Input: part model. Units: mm. Frame: model coordinates. A direction names the side the tool comes from. Coordinates: 2 decimals unless noted, no trailing zeros. Order: outer loops, then holes, each group sorted by start corner. A loop starts at its lowest first (then second) coordinate and runs counter-clockwise, first axis right, second up. Notation, with made-up numbers: (58, 47.5) -> (96, 47.5) arc R23 ccw to (96, 77.5) -> close; hole circle Ø7 at (24.5, 84). An arc over 180 degrees is marked (long way). Use one line per item in the form item = value. Start each with the question number.
1) Section query C-C on x = 8. Output: boundary loops of the cut face in (y, z).
2) Access query for faces 4 (the flat face through (25, -10, 17)), 5 (the flat face through (-48, 12, 10)), 6 (the flat face through (-62, -12, 2)), 7 (the flat face through (-31, -33, 71)), 8 (the flat face through (-46.22, -25.416, 19.564)). Directions: +Z, -Z, +X, -X, +Y, -Y. A direction counts if a zero-diameter tool reaches every point of the face in a straight line with its end or side. Return the directions, or none.
3) Draft query along X for faces 1 (the flat face through (-62, -19.5, 75)), 2 (the flat face through (-29, -33, 71)), 3 (the flat face through (-78.73, 3.11, 20.14)). Return one class per face: pulls with the +X half, pulls with the -X half, needs draft (parallel to the pull), parting line crosses it, or undercut.
4) Section query A-A on y = 8. Output: boundary loops of the cut face in (x, z).
5) Section query B-B on y = -8. Output: boundary loops of the cut face in (x, z), then the cut area to 3 significant figures.
6) Ray query, line 1 along Y through (x, z) = (0, 27); line 2 along X through (y, z) = (0.5, 56); line 3 along X through (y, z) = (-8, 4). Return the intervals inside material, ascending.
7) Pin query (flat end, axial travel): pin 1 (1.1 mm diameter, centred on y = -34, z = 11, fed in from +X); pin 2 (10 mm diameter, centred on x = 7.5, y = -12, fed in from +Z); pin 3 (13 mm diameter, centred on y = -7.5, z = 65.5, fed in from +X); pin 4 (2.5 mm diameter, centred on x = 8, y = 0, fed in from -Z). Return the tip coordinate at first contact, or that it passes through.
8) Section query D-D on y = -16. Output: boundary loops of the cut face in (x, z).
from build123d import *
from build123d.topology import SkipClean

# Parameters (mm, degrees)
SKETCH_1_W            = 50
SKETCH_1_H            = 35
EXTRUDE_1_DEPTH       = 10
HOLE_WIZARD_370_D     = 10.5
HOLE_WIZARD_475_D     = 3.2
SKETCH_6_W            = 10
SKETCH_6_H            = 52
EXTRUDE_2_DEPTH       = 70
EXTRUDE_3_DEPTH       = 52
SKETCH_10_W           = 30
SKETCH_10_H           = 15
SKETCH_10_H_2         = 7
CUT_EXTRUDE_1_DEPTH   = 66
SKETCH_12_W           = 5
SKETCH_12_H           = 15
EXTRUDE_4_DEPTH       = 2
EXTRUDE_5_DEPTH       = 10
RIB_6_REACH           = 107.429
SKETCH_15_WALL_W      = 243.090204886
SKETCH_15_WALL_H      = 10
SKETCH_16_W           = 10
SKETCH_16_H           = 10
EXTRUDE_6_DEPTH       = 17
FILLET_1_RADIUS       = 5
FILLET_1_LENGTH       = 10
CUT_EXTRUDE_3_DEPTH   = 3
EXTRUDE_8_DEPTH       = 2
FILLET_3_R            = 1
SKETCH_20_R           = 5
CUT_EXTRUDE_4_DEPTH   = 106.654483654
CHAMFER_3_SIZE        = 3
SKETCH_22_R           = 1.6
SKETCH_22_R_2         = 4.65
SKETCH_22_R_3         = 5.25
EXTRUDE_9_DEPTH       = 74
EXTRUDE_10_DEPTH      = 49
SKETCH_25_W           = 30
SKETCH_25_H           = 15
CUT_EXTRUDE_5_DEPTH   = 66
SKETCH_26_R           = 12.5
CUT_EXTRUDE_6_DEPTH   = 50
SKETCH_27_W           = 25
SKETCH_27_H           = 70.37051412
SKETCH_27_W_2         = 27.110275364
CUT_EXTRUDE_7_DEPTH   = 50
SKETCH_28_R           = 5
CUT_EXTRUDE_8_DEPTH   = 132.601177488
MIRROR_2_COPY_1_DEPTH = 2


with BuildPart() as part:
    # 草图1 → 凸台-拉伸1 (new body)
    with BuildSketch(Plane.XY):
        Rectangle(SKETCH_1_W, SKETCH_1_H)
    extrude(amount=EXTRUDE_1_DEPTH)

    # Hole Wizard 370 (through all)
    with Locations(Plane.XY.offset(10)):
        with Locations((0, 0)):
            Hole(HOLE_WIZARD_370_D / 2)

    # Hole Wizard 475 (through all)
    with Locations(Plane.XY.offset(10)):
        with Locations((8, 0), (0, 8), (-8, 0), (0, -8)):
            Hole(HOLE_WIZARD_475_D / 2)

    # 草图6 → 凸台-拉伸2 (add)
    with BuildSketch(Plane.ZY.offset(25)):
        with Locations((5, -8.5)):
            Rectangle(SKETCH_6_W, SKETCH_6_H)
    extrude(amount=EXTRUDE_2_DEPTH)

    # 草图9 → 凸台-拉伸3 (add, through all)
    with BuildSketch(Plane(origin=(0, 17.5, 0), x_dir=(1, 0, 0), z_dir=(0, 1, 0))):
        Polygon((-95, -30), (-62, -10), (-95, -10), align=None)
        Polygon((-29, -30), (-29, -10), (-62, -10), align=None)
    extrude(amount=-EXTRUDE_3_DEPTH)

    # 草图10 → 切除-拉伸1 (cut)
    with BuildSketch(Plane.ZY.offset(95)):
        with Locations((15, -12)):
            Rectangle(SKETCH_10_W, SKETCH_10_H)
        with Locations((15, 14)):
            Rectangle(SKETCH_10_W, SKETCH_10_H_2)
    extrude(amount=-CUT_EXTRUDE_1_DEPTH, mode=Mode.SUBTRACT)

    # 草图12 → 凸台-拉伸4 (add)
    with BuildSketch(Plane(origin=(0, 0, 0), x_dir=(-1, 0, 0), z_dir=(0, 0, -1))):
        with Locations((85.5, -12)):
            Rectangle(SKETCH_12_W, SKETCH_12_H)
        with Locations((39.5, -12)):
            Rectangle(SKETCH_12_W, SKETCH_12_H)
        with Locations((62.5, -12)):
            Rectangle(SKETCH_12_W, SKETCH_12_H)
    extrude(amount=-EXTRUDE_4_DEPTH)

    # 草图14 → 凸台-拉伸5 (add)
    with BuildSketch(Plane(origin=(0, 0, 0), x_dir=(-1, 0, 0), z_dir=(0, 0, -1))):
        Polygon((95, 10.5), (29, 17.5), (29, 10.5), align=None)
    extrude(amount=-EXTRUDE_5_DEPTH)

    # 草图15 wall → 筋6 (add, up to next)
    with BuildSketch(Plane(origin=(-12.5, -26, 0), x_dir=(0.82692650207, 0.562310021407, 0), z_dir=(0.562310021407, -0.82692650207, 0)), mode=Mode.PRIVATE) as rib_6_sk1:
        with Locations((0, 5)):
            Rectangle(SKETCH_15_WALL_W, SKETCH_15_WALL_H)
    rib_6_tool1 = extrude(rib_6_sk1.sketch, amount=-RIB_6_REACH, mode=Mode.PRIVATE) - part.part
    add(rib_6_tool1.solids().sort_by_distance((-12.5, -26, 0))[0])

    # 草图16 → 凸台-拉伸6 (add)
    with BuildSketch(Plane.XZ.offset(17.5)):
        with Locations((20, 5)):
            Rectangle(SKETCH_16_W, SKETCH_16_H)
    extrude(amount=EXTRUDE_6_DEPTH)

    # 圆角1: full round fillet: the end face becomes a half cylinder, R = half its width
    fillet_1_face = Plane((20, -34.5, 5), x_dir=(-1, 0, 0), z_dir=(0, -1, 0))  # on the end face: x along it, z out of the body
    fillet_1_slab = fillet_1_face.offset(-FILLET_1_RADIUS / 2) * Box(FILLET_1_LENGTH, 2 * FILLET_1_RADIUS, FILLET_1_RADIUS, mode=Mode.PRIVATE)  # the body's end, R deep
    fillet_1_round = Plane((20, -29.5, 5), x_dir=(0, -1, 0), z_dir=(-1, 0, 0)) * Cylinder(FILLET_1_RADIUS, FILLET_1_LENGTH, mode=Mode.PRIVATE)  # its axis R under the face
    add(fillet_1_slab - fillet_1_round, mode=Mode.SUBTRACT)

    # 草图17 → 切除-拉伸3 (cut)
    with BuildSketch(Plane.XZ.offset(34.5)):
        Polygon((-95, 30), (-62, 10), (-29, 30), (-29, 10), (-17.881583213, 10), (-17.881583213, 0), (-29, 0), (-95, 0), align=None)
    extrude(amount=-CUT_EXTRUDE_3_DEPTH, mode=Mode.SUBTRACT)

    # 草图19 → 凸台-拉伸8 (add)
    with BuildSketch(Plane.ZY.offset(95)):
        with BuildLine():
            Line((25.690911714, -31.5), (0, -31.5))
            ThreePointArc((0, -31.5), (12.845455857, -35.183375195), (25.690911714, -31.5))
        make_face()
    extrude_8 = extrude(amount=-EXTRUDE_8_DEPTH)

    # 圆角3
    fillet_3_edges = [part.edges().sort_by_distance(p)[0] for p in [
        (-95, -25.5, 30),
        (-95, -31.5, 27.845455857),
        (-78.5, -31.5, 20),
    ]]
    fillet(fillet_3_edges, radius=FILLET_3_R)

    # 草图20 → 切除-拉伸4 (cut, through all)
    with BuildSketch(Plane(origin=(0, 0, 0), x_dir=(-1, 0, 0), z_dir=(0, 0, -1))):
        with Locations((20, 0)):
            Circle(SKETCH_20_R)
    extrude(amount=-CUT_EXTRUDE_4_DEPTH, mode=Mode.SUBTRACT)

    # 倒角3
    # the kernel refuses this chamfer: 3 mm, written as the material it takes off along each edge
    with BuildSketch(Plane(origin=(25, 17.5, -7.715048964), x_dir=(0.02749587661058678, -0.9996219169112968, 0), z_dir=(0, 0, 1))) as chamfer_3_piece_1:
        Polygon((CHAMFER_3_SIZE * 0.999621916911, -CHAMFER_3_SIZE * 0.0274958766106), (-CHAMFER_3_SIZE * 0.0274958766106, -CHAMFER_3_SIZE * 0.999621916911), (0, 0), align=None)
    extrude(amount=25.430097928, mode=Mode.SUBTRACT)
    with BuildSketch(Plane(origin=(-95, 18.215048964, 0), x_dir=(0.9996219169112968, 0, -0.02749587661058636), z_dir=(0, -1, 0))) as chamfer_3_piece_2:
        Polygon((CHAMFER_3_SIZE * 0.999621916911, CHAMFER_3_SIZE * 0.0274958766106), (-CHAMFER_3_SIZE * 0.0274958766106, CHAMFER_3_SIZE * 0.999621916911), (0, 0), align=None)
    extrude(amount=30.430097928, mode=Mode.SUBTRACT)
    with BuildSketch(Plane(origin=(-95, -11.784951036, 0), x_dir=(-0.027495876610586778, 0, 0.9996219169112968), z_dir=(0, -1, 0))) as chamfer_3_piece_3:
        Polygon((CHAMFER_3_SIZE * 0.999621916911, -CHAMFER_3_SIZE * 0.0274958766106), (-CHAMFER_3_SIZE * 0.0274958766106, -CHAMFER_3_SIZE * 0.999621916911), (0, 0), align=None)
    extrude(amount=27.430097928, mode=Mode.SUBTRACT)

    # 草图22 → 凸台-拉伸9 (add)
    with SkipClean():  # the faces are left unmerged after this step: merging them gives an invalid solid
        with BuildSketch(Plane.XY.offset(10)):
            Polygon((-29, 17.5), (-29, -31.5), (-20.588235294, -31.5), (0, -17.5), (15, -17.5), (15, -29.5), (25, -29.5), (25, 14.5), (22, 17.5), align=None)
            with Locations((0, -8)):
                Circle(SKETCH_22_R, mode=Mode.SUBTRACT)
            with Locations((0, 8)):
                Circle(SKETCH_22_R, mode=Mode.SUBTRACT)
            with Locations((8, 0)):
                Circle(SKETCH_22_R, mode=Mode.SUBTRACT)
            with Locations((-8, 0)):
                Circle(SKETCH_22_R, mode=Mode.SUBTRACT)
            with Locations((-20, 0)):
                Circle(SKETCH_22_R_2, mode=Mode.SUBTRACT)
            Circle(SKETCH_22_R_3, mode=Mode.SUBTRACT)
        extrude(amount=EXTRUDE_9_DEPTH)
    add(part.part.scale(1), mode=Mode.REPLACE)  # the faces are merged on a copy

    # 草图24 → 凸台-拉伸10 (add)
    with SkipClean():  # the faces are left unmerged after this step: merging them gives an invalid solid
        with BuildSketch(Plane(origin=(0, 17.5, 0), x_dir=(1, 0, 0), z_dir=(0, 1, 0))):
            Polygon((-95, -74), (-95, -54), (-62, -74), (-29, -54), (-29, -74), (-29, -84), (-95, -84), align=None)
        extrude(amount=-EXTRUDE_10_DEPTH)

    # 草图25 → 切除-拉伸5 (cut)
    with SkipClean():  # the faces are left unmerged after this step: merging them gives an invalid solid
        with BuildSketch(Plane.ZY.offset(95)):
            with Locations((69, -12)):
                Rectangle(SKETCH_25_W, SKETCH_25_H)
        extrude(amount=-CUT_EXTRUDE_5_DEPTH, mode=Mode.SUBTRACT)

    # 草图26 → 切除-拉伸6 (cut)
    with BuildSketch(Plane.XY.offset(84)):
        Circle(SKETCH_26_R)
    extrude(amount=-CUT_EXTRUDE_6_DEPTH, mode=Mode.SUBTRACT)

    # 草图27 → 切除-拉伸7 (cut)
    with BuildSketch(Plane.XY.offset(84)):
        Rectangle(SKETCH_27_W, SKETCH_27_H)
        with Locations((26.055137682, 0)):
            Rectangle(SKETCH_27_W_2, SKETCH_27_H)
    extrude(amount=-CUT_EXTRUDE_7_DEPTH, mode=Mode.SUBTRACT)

    # 镜向1: 凸台-拉伸8 across plane
    add(extrude_8.mirror(Plane(origin=(0, 0, 42), x_dir=(1, 0, 0), z_dir=(0, 0, -1))))

    # 草图28 → 切除-拉伸8 (cut, through all)
    with BuildSketch(Plane.XY.offset(84)):
        with Locations(Location((-20, 0, 0), (0, 0, 180))):
            Circle(SKETCH_28_R)
    extrude(amount=-CUT_EXTRUDE_8_DEPTH, mode=Mode.SUBTRACT)

    # 镜向2: 凸台-拉伸8 across plane
    add(extrude_8.mirror(Plane.ZY.offset(62)))

    # 镜向2 copy 1 sketch → 镜向2 copy 1 (add)
    with BuildSketch(Plane(origin=(-29, 0, 84), x_dir=(0, 0, -1), z_dir=(1, 0, 0))):
        with BuildLine():
            Line((25.690911714, -31.5), (0, -31.5))
            ThreePointArc((0, -31.5), (12.845455857, -35.183375195), (25.690911714, -31.5))
        make_face()
    extrude(amount=-MIRROR_2_COPY_1_DEPTH)


solid = part.part
Answers below:
q1.outline = (-17.5, 0) -> (-1.6, 0) -> (-1.6, 34) -> (-17.5, 34) -> close; (1.6, 0) -> (17.5, 0) -> (17.5, 34) -> (1.6, 34) -> close
q2.face_4 = +Z, -Z, +X, +Y, -Y
q2.face_5 = -X, +Y
q2.face_6 = +Z, -X
q2.face_7 = +Z, -Z, -Y
q2.face_8 = +Y, -Y
q3.face_1 = needs draft
q3.face_2 = pulls with the +X half
q3.face_3 = undercut
q4.outline = (-95, 3) -> (-92, 0) -> (-1.6, 0) -> (-1.6, 34) -> (-12.5, 34) -> (-12.5, 84) -> (-95, 84) -> (-95, 54) -> (-62, 74) -> (-29, 54) -> (-29, 30) -> (-62, 10) -> (-95, 30) -> close; (1.6, 0) -> (25, 0) -> (25, 34) -> (1.6, 34) -> close
q5.outline = (-88, 0) -> (-83, 0) -> (-83, 2) -> (-88, 2) -> close; (-65, 0) -> (-60, 0) -> (-60, 2) -> (-65, 2) -> close; (-42, 0) -> (-37, 0) -> (-37, 2) -> (-42, 2) -> close; (-29, 0) -> (-1.6, 0) -> (-1.6, 34) -> (-12.5, 34) -> (-12.5, 84) -> (-29, 84) -> close; (1.6, 0) -> (25, 0) -> (25, 34) -> (1.6, 34) -> close
q5.area = 2,580 mm^2
q6.line_1 = -17.5 to -9.6, -6.4 to -5.25, 5.25 to 6.4, 9.6 to 17.5
q6.line_2 = -95 to -91.7, -32.3 to -24.97, -15.03 to -12.5
q6.line_3 = -29 to -1.6, 1.6 to 25
q7.pin_1 = -29
q7.pin_2 = 34
q7.pin_3 = -12.5
q7.pin_4 = through
q8.outline = (-88, 0) -> (-83, 0) -> (-83, 2) -> (-88, 2) -> close; (-65, 0) -> (-60, 0) -> (-60, 2) -> (-65, 2) -> close; (-42, 0) -> (-37, 0) -> (-37, 2) -> (-42, 2) -> close; (-29, 0) -> (25, 0) -> (25, 34) -> (-12.5, 34) -> (-12.5, 84) -> (-29, 84) -> close
